```python
from build123d import *

# Parameters (mm, degrees)
SKETCH1_R           = 10
SKETCH1_W           = 50.8
SKETCH1_H           = 19.05
BOSS_EXTRUDE1_DEPTH = 19.05


with BuildPart() as part:
    # Sketch1 → Boss-Extrude1 (new body)
    with BuildSketch(Plane(origin=(0, 0, 0), x_dir=(1, 0, 0), z_dir=(0, 1, 0))):
        with BuildLine():
            Line((-25.4, 0), (-25.4, 711.2))
            Line((-25.4, 711.2), (101.6, 711.2))
            Line((101.6, 711.2), (152.4, 457.2))
            Line((152.4, 457.2), (25.4, 0))
            ThreePointArc((25.4, 0), (0, -25.4), (-25.4, 0))
        make_face()
        Circle(SKETCH1_R, mode=Mode.SUBTRACT)
        with Locations((76.2, 457.2)):
            Rectangle(SKETCH1_W, SKETCH1_H, mode=Mode.SUBTRACT)
    extrude(amount=BOSS_EXTRUDE1_DEPTH)


solid = part.part
```
Check sheet for the modelled part. Datum: model origin and axes. Units: mm. A direction names the side the tool comes from. Give positions to 0.01 mm unless a question says otherwise; leave off trailing zeros. Order: outer loops, then holes, each group sorted by start corner. A loop starts at its lowest first (then second) coordinate and runs counter-clockwise, first axis right, second up. Notation, with made-up numbers: M 19,-13.75 L 63,-13.75 A32 cw 63,17.25 Z; hole C 39,15.5 d10. An arc over 180 degrees is marked long. Answer in a Markdown table with one row per item.
1) Cross-section at A-A, the plane y = 4.75. Enter the section's corners in (x, z) (3 decimals).
Filled sheet:
| item | result |
|---|---|
| outline | M -25.4,-711.2 L 101.6,-711.2 L 152.4,-457.2 L 25.4,0 A25.4 ccw -25.4,0 Z; hole C 0,0 d20; hole M 50.8,-466.725 L 101.6,-466.725 L 101.6,-447.675 L 50.8,-447.675 Z |
2) Access from +Z, -Z, +X, -X, +Y, -Y to the whole of each face (thin tool, end or side, straight path). Record for faces 1 (the flat face through (101.6, 9, -457)), 2 (the flat face through (89.79, 9.39, -231.8)).
Filled sheet:
| item | result |
|---|---|
| face 1 | +Y, -Y |
| face 2 | +Z, +X, +Y, -Y |
3) Release check for a two-part mould opening along X. For faces 3 (the flat face through (76, 9, -447.675)), 4 (the cylindrical face through (0.559, 9.392, 25.394)), 5 (the flat face through (45, 0, -430)) record: +X half, -X half, draft (parallel to the pull), parting line (faces both ways), or undercut.
Filled sheet:
| item | result |
|---|---|
| face 3 | undercut |
| face 4 | parting line |
| face 5 | draft |
4) Cross-section at C-C, the plane x = 95.5. Enter the section's corners in (y, z) (3 decimals).
Filled sheet:
| item | result |
|---|---|
| outline | M 0,-711.2 L 19.05,-711.2 L 19.05,-466.725 L 0,-466.725 Z; M 0,-447.675 L 19.05,-447.675 L 19.05,-252.36 L 0,-252.36 Z |
5) Cross-section at D-D, the plane z = -238.5. Enter the section's corners in (x, y).
Filled sheet:
| item | result |
|---|---|
| outline | M -25.4,0 L 91.65,0 L 91.65,19.05 L -25.4,19.05 Z |
6) Gauge pin test, flat ends, axial feed: P1, Ø16, axis at x = 0, z = 0, coming from the +Y side; P2, Ø1, axis at y = 5.5, z = -378, coming from the +X side; P3, Ø8, axis at y = 14, z = -151, coming from the +X side; P4, Ø10, axis at y = 15.5, z = -430.5, coming from the +X side. Record the tip position at first contact, or that the pin passes through.
Filled sheet:
| item | result |
|---|---|
| P1 | passes through |
| P2 | stops at x = 130.54 |
| P3 | stops at x = 68.46 |
| P4 | stops at x = 146.37 |
7) Thickness scan on L1, parallel to Z at x = 0, y = 11; L2, parallel to X at y = 3.5, z = -454; L3, parallel to X at y = 11, z = -16. Record the ranges inside material, lowest first. Write a range as [from, to].
Filled sheet:
| item | result |
|---|---|
| L1 | z = [-711.2, -10], [10, 25.4] |
| L2 | x = [-25.4, 50.8], [101.6, 151.51] |
| L3 | x = [-25.4, 29.84] |
8) Cross-section at B-B, the plane x = 0. Enter the section's corners in (y, z), plus the area to 3 significant figures.
Filled sheet:
| item | result |
|---|---|
| outline | M 0,-711.2 L 19.05,-711.2 L 19.05,-10 L 0,-10 Z; M 0,10 L 19.05,10 L 19.05,25.4 L 0,25.4 Z |
| area | 13,700 mm2 |
